Part model, mm, in its own coordinate system. Give positions to 0.01 mm unless a question says otherwise; leave off trailing zeros. Write each loop counter-clockwise with the first axis right and the second up, starting at its lowest first coordinate (ties: lowest second). Pieces come first, ordered by that corner, then holes.
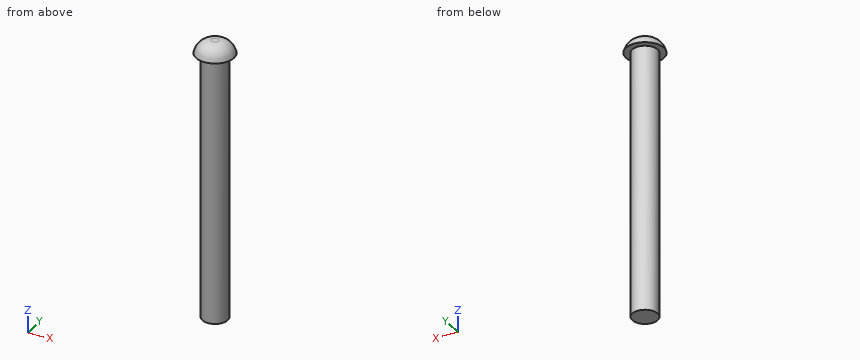
Autodesk Inventor part; units mm, degrees
ref_plane "YZ Plane" through (0, 0, 0) normal (1, 0, 0) x (0, 1, 0)
ref_plane "XZ Plane" through (0, 0, 0) normal (0, 1, 0) x (-1, 0, 0)
ref_plane "XY Plane" through (0, 0, 0) normal (0, 0, 1) x (1, 0, 0)
sketch "Sketch1" plane through (0, 0, 0) normal (0, 0, 1) x (1, 0, 0)
  circle A0 centre (0, 0) radius 2.54
  dimension "d0" = 5.08
extrude "Extrusion1" add sketch "Sketch1" along normal blind 53.34
sketch "Sketch2" plane through (0, 0, 53.34) normal (0, 0, 1) x (1, 0, 0)
  circle A0 centre (0, 0) radius 2.54
  circle A1 centre (0, 0) radius 3.81
  dimension "d3" = 7.62
extrude "Extrusion2" add sketch "Sketch2" along normal blind 2.54 contours A0 | A1
fillet "Fillet1" radius 3.175 1 edges at (-3.81, 0, 55.88)
properties part number "HingeBolt"
1) Wall check: L1, parallel to Y at x = 0, z = 7; L2, parallel to Z at x = 1, y = -2.5; L3, parallel to Z at x = 1, y = -2.25. Give the ranges that are in metal, low to high.
Answers follow:
L1: y = -2.54 to 2.54
L2: z = 53.34 to 55.18
L3: z = 0 to 55.35
2) Saw through at A-A, the plane z = 44. Write the cut outline in (x, y), then the cut area to 3 significant figures.
Answers follow:
outline: circle Ø5.08 at (0, 0)
area: 20.3 mm2
3) Pin check, flat tips, straight feed: pin 1 Ø3 at (y, z) = (0, 19) entering from +X; pin 2 Ø1 at (x, z) = (2.5, 11) entering from -Y; pin 3 Ø1 at (y, z) = (2.5, 15) entering from +X. Stop position of each tip, or through.
Answers follow:
pin 1: stops at x = 2.54
pin 2: stops at y = -1.57
pin 3: stops at x = 1.57
